Geometry: final body of the model. Coordinates: model frame, mm. Coordinates: 2 decimals unless noted, no trailing zeros. Write each loop counter-clockwise with the first axis right and the second up, starting at its lowest first coordinate (ties: lowest second). Pieces come first, ordered by that corner, then holes. Notation, with made-up numbers: (6, 54) - (52, 54) arc R9 cw to (52, 64) - close; hole circle Ø4 at (-22.5, -25). An arc over 180 degrees is marked (long way). Answer as a JSON object with one key per item and string values. Group by question number.
Item 1: Section A-A on y = 128.5. Return loops of the section in (x, z).
Item 2: Section B-B on z = 5. Return loops of the section in (x, y).
Item 3: First-contact query: pin 1 Ø3 at (x, z) = (118.5, 18.5) entering from -Y; pin 2 Ø12 at (x, z) = (174.5, 13) entering from +Y; pin 3 Ø1 at (x, z) = (254.5, 15) entering from -Y. Flat tips, straight axial feed; report the tip coordinate or a pass-through.
Item 4: Section C-C on x = 69.5. Return loops of the section in (y, z), and give its area (3 significant figures).
Item 5: Section D-D on x = -44. Return loops of the section in (y, z), and give its area (3 significant figures).
Item 6: Line query: line 1 along X through (y, z) = (465, 5.75); line 2 along Y through (x, z) = (202, 6.25) (3 decimals); line 3 along Y through (x, z) = (219, 23.75). Output: solid intervals per line, ascending. Write a range as from..to.
```python
from build123d import *

# Parameters (mm, degrees)
F1_DEPTH = 25


with BuildPart() as f1:
    # F0 (on Top) → F1 (new body)
    with BuildSketch(Plane.XY):
        with BuildLine():
            Line((-88.936575, 490.166194), (-88.936575, -209.833806))
            Line((-88.936575, -209.833806), (-28.936575, -209.833806))
            ThreePointArc((-28.936575, -209.833806), (211.063425, 30.166194), (451.063425, -209.833806))
            Line((451.063425, -209.833806), (511.063425, -209.833806))
            Line((511.063425, -209.833806), (511.063425, 490.166194))
            ThreePointArc((511.063425, 490.166194), (423.19546, 702.298228), (211.063425, 790.166194))
            ThreePointArc((211.063425, 790.166194), (-1.068609, 702.298228), (-88.936575, 490.166194))
        make_face()
        with BuildLine():
            ThreePointArc((0, 490.166194), (62.434461, 635.647461), (211.063425, 690.166194))
            ThreePointArc((211.063425, 690.166194), (357.637827, 634.46583), (418.990907, 490.166194))
            Line((418.990907, 490.166194), (418.990907, 0))
            ThreePointArc((418.990907, 0), (209.495453, 72.209681), (0, 0))
            Line((0, 0), (0, 490.166194))
        make_face(mode=Mode.SUBTRACT)
    extrude(amount=F1_DEPTH)


solid = f1.part
```
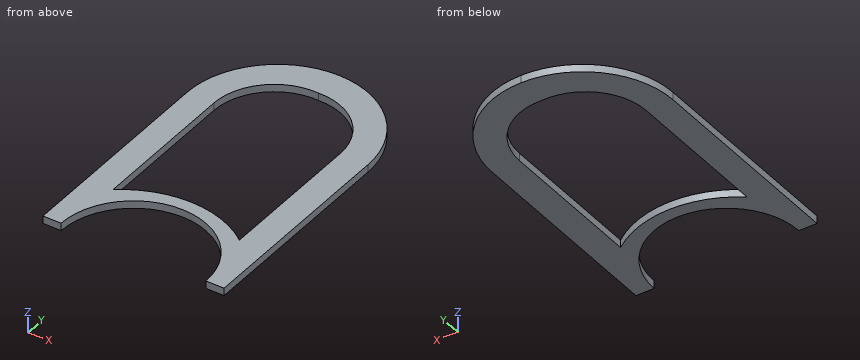
Checks:
{
 "1": {"outline": "(-88.94, 0) - (0, 0) - (0, 25) - (-88.94, 25) - close; (418.99, 0) - (511.06, 0) - (511.06, 25) - (418.99, 25) - close"},
 "2": {"outline": "(-88.94, -209.83) - (-28.94, -209.83) arc R240 cw to (451.06, -209.83) - (511.06, -209.83) - (511.06, 490.17) arc R300 ccw to (211.06, 790.17) arc R300 ccw to (-88.94, 490.17) - close; hole (0, 0) arc R340 cw to (418.99, 0) - (418.99, 490.17) arc R200 ccw to (211.06, 690.17) arc R200 ccw to (0, 490.17) - close"},
 "3": {"pin 1": "y = 10.96", "pin 2": "y = 788.61", "pin 3": "y = 26.11"},
 "4": {"outline": "(-16.03, 0) - (42.05, 0) - (42.05, 25) - (-16.03, 25) - close; (642.03, 0) - (754.67, 0) - (754.67, 25) - (642.03, 25) - close", "area": "4,270 mm^2"},
 "5": {"outline": "(-209.83, 0) - (648.1, 0) - (648.1, 25) - (-209.83, 25) - close", "area": "21,400 mm^2"},
 "6": {"line 1": "-88.94..0, 418.99..511.06", "line 2": "29.995..72.127, 690.462..790.029", "line 3": "30.03..72.08, 690.32..790.06"}
}
